Build history of the part. All positions in model axes, mm. Face numbers are marked on the shaded views. Coordinates: 2 decimals unless noted, no trailing zeros. Write each loop counter-clockwise with the first axis right and the second up, starting at its lowest first coordinate (ties: lowest second). Pieces come first, ordered by that corner, then holes.
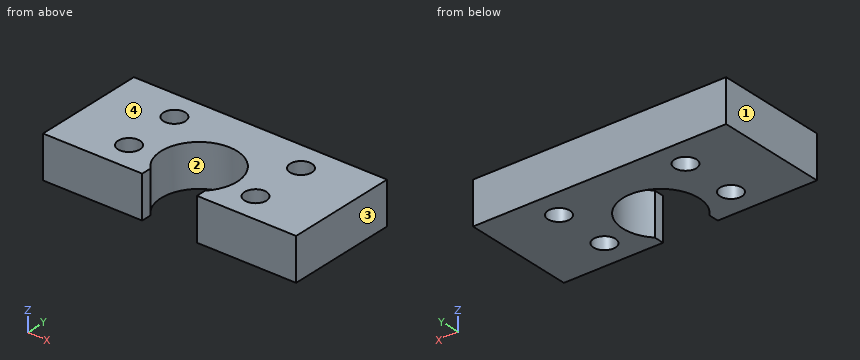
```python
from build123d import *

# Parameters (mm, degrees)
SZKIC1_W                    = 36
SZKIC1_H                    = 16
DODANIE_WYCI_GNI_CIE1_DEPTH = 6
WYTNIJ_WYCI_GNI_CIE1_DEPTH  = 6
SZKIC3_R                    = 1.55
WYTNIJ_WYCI_GNI_CIE2_DEPTH  = 74.51650454


with BuildPart() as part:
    # Szkic1 → Dodanie-wyciągnięcie1 (new body)
    with BuildSketch(Plane.XY):
        with Locations((53.502982034, -8)):
            Rectangle(SZKIC1_W, SZKIC1_H)
    extrude(amount=-DODANIE_WYCI_GNI_CIE1_DEPTH)

    # Szkic2 → Wytnij-wyciągnięcie1 (cut)
    with BuildSketch(Plane.XY):
        with BuildLine():
            Line((49.612982034, -14.93), (49.612982034, -16))
            Line((49.612982034, -16), (57.392982034, -16))
            Line((57.392982034, -16), (57.392982034, -14.93))
            Line((57.392982034, -14.93), (57.392982034, -14.545383825))
            ThreePointArc((57.392982034, -14.545383825), (53.502982034, -5.4), (49.612982034, -14.545383825))
            Line((49.612982034, -14.545383825), (49.612982034, -14.93))
        make_face()
    extrude(amount=-WYTNIJ_WYCI_GNI_CIE1_DEPTH, mode=Mode.SUBTRACT)

    # Szkic3 → Wytnij-wyciągnięcie2 (cut, through all)
    with BuildSketch(Plane(origin=(0, 0, -6), x_dir=(-1, 0, 0), z_dir=(0, 0, -1))):
        with Locations((-44.502982034, -12)):
            Circle(SZKIC3_R)
        with Locations((-44.502982034, -4)):
            Circle(SZKIC3_R)
        with Locations((-62.502982034, -12)):
            Circle(SZKIC3_R)
        with Locations((-62.502982034, -4)):
            Circle(SZKIC3_R)
    extrude(amount=-WYTNIJ_WYCI_GNI_CIE2_DEPTH, mode=Mode.SUBTRACT)


solid = part.part
```
1. Saw through at C-C on y = -12. List the corners of the cut face in (x, z), plus the area to 3 significant figures.
Computed values:
outline: (35.5, -6) - (42.95, -6) - (42.95, 0) - (35.5, 0) - close; (46.05, -6) - (48.24, -6) - (48.24, 0) - (46.05, 0) - close; (58.77, -6) - (60.95, -6) - (60.95, 0) - (58.77, 0) - close; (64.05, -6) - (71.5, -6) - (71.5, 0) - (64.05, 0) - close
area: 116 mm2
2. Saw through at B-B on z = -2.65. List the corners of the cut face in (x, y).
Computed values:
outline: (35.5, -16) - (49.61, -16) - (49.61, -14.55) arc R5.4 cw (long way) to (57.39, -14.55) - (57.39, -16) - (71.5, -16) - (71.5, 0) - (35.5, 0) - close; hole circle Ø3.1 at (44.5, -12); hole circle Ø3.1 at (44.5, -4); hole circle Ø3.1 at (62.5, -12); hole circle Ø3.1 at (62.5, -4)
3. Mould opens along X. For the marked faces 1, 2, 3 and 4 say: +X half, -X half, draft (parallel to the pull), parting line (faces both ways), or undercut.
Computed values:
face 1: -X half
face 2: undercut
face 3: +X half
face 4: draft
4. Probe line 1 along X through (y, z) = (-5, -0.5); line 2 along X through (y, z) = (-10.8, -3.4); line 3 along X through (y, z) = (-3.5, -0.7). List the from-to ranges inside material, lowest first.
Computed values:
line 1: x = 35.5 to 43.32, 45.69 to 61.32, 63.69 to 71.5
line 2: x = 35.5 to 43.52, 45.48 to 48.1, 58.9 to 61.52, 63.48 to 71.5
line 3: x = 35.5 to 43.04, 45.97 to 61.04, 63.97 to 71.5
5. Saw through at D-D on y = -7.75. List the corners of the cut face in (x, z), plus the area to 3 significant figures.
Computed values:
outline: (35.5, -6) - (49.05, -6) - (49.05, 0) - (35.5, 0) - close; (57.96, -6) - (71.5, -6) - (71.5, 0) - (57.96, 0) - close
area: 163 mm2
6. Saw through at A-A on y = -4. List the corners of the cut face in (x, z).
Computed values:
outline: (35.5, -6) - (42.95, -6) - (42.95, 0) - (35.5, 0) - close; (46.05, -6) - (60.95, -6) - (60.95, 0) - (46.05, 0) - close; (64.05, -6) - (71.5, -6) - (71.5, 0) - (64.05, 0) - close
